```python
from build123d import *

# Parameters (mm, degrees)
SKETCH1_W           = 6
SKETCH1_H           = 20
SKETCH1_R           = 2
BOSS_EXTRUDE1_DEPTH = 3
SKETCH4_R           = 1.5
CUT_EXTRUDE1_DEPTH  = 10
SKETCH5_W           = 0.8
SKETCH5_H           = 4.49496607
CUT_EXTRUDE2_DEPTH  = 7
SKETCH6_R           = 1
CUT_EXTRUDE3_DEPTH  = 7


with BuildPart() as part:
    # Sketch1 → Boss-Extrude1 (new body, symmetric)
    with BuildSketch(Plane.XY):
        with Locations((0, 195)):
            Rectangle(SKETCH1_W, SKETCH1_H)
        with Locations((0, 200)):
            Circle(SKETCH1_R, mode=Mode.SUBTRACT)
    extrude(amount=BOSS_EXTRUDE1_DEPTH, both=True)

    # Sketch3 → Cut-Revolve3 (revolve, cut)
    with BuildSketch(Plane.XY):
        Polygon((-3, 185), (-2.3, 185), (-3, 188.032033112), (-6.917363823, 205), (-6.917363823, 185), align=None)
    revolve(axis=Axis((0, 200, 0), (0, -1, 0)), mode=Mode.SUBTRACT)

    # Sketch4 → Cut-Extrude1 (cut)
    with BuildSketch(Plane.XZ.offset(-185)):
        Circle(SKETCH4_R)
    extrude(amount=-CUT_EXTRUDE1_DEPTH, mode=Mode.SUBTRACT)

    # Sketch5 → Cut-Extrude2 (cut, through all)
    with BuildSketch(Plane.XY.offset(3)):
        with Locations((0, 202.752516965)):
            Rectangle(SKETCH5_W, SKETCH5_H)
    extrude(amount=-CUT_EXTRUDE2_DEPTH, mode=Mode.SUBTRACT)

    # Sketch6 → Cut-Extrude3 (cut, through all)
    with BuildSketch(Plane(origin=(3, 0, 0), x_dir=(0, 0, -1), z_dir=(1, 0, 0))):
        with Locations((0, 203)):
            Circle(SKETCH6_R)
    extrude(amount=-CUT_EXTRUDE3_DEPTH, mode=Mode.SUBTRACT)


solid = part.part
```
The listing builds one solid part. Answer for the finished solid, in the listing's coordinates (mm). A direction names the side the tool comes from. Give positions to 0.01 mm unless a question says otherwise; leave off trailing zeros. Order: outer loops, then holes, each group sorted by start corner. A loop starts at its lowest first (then second) coordinate and runs counter-clockwise, first axis right, second up.
1) Consider line 1 along Z through (x, y) = (1.9, 203); line 2 along Z through (x, y) = (0, 191.25); line 3 along X through (y, z) = (200, 0.35). Determine where each line is inside the solid, lowest interval first.
Reported:
line 1: z = -3 to -1, 1 to 3
line 2: z = -3 to -1.5, 1.5 to 3
line 3: x = -3 to -2, 2 to 3
2) Find section A-A on y = 203. Write down the section's boundary in (x, z), then the cut area to 3 significant figures.
Reported:
outline: (-3, -3) - (-0.4, -3) - (-0.4, -1) - (-3, -1) - close; (-3, 1) - (-0.4, 1) - (-0.4, 3) - (-3, 3) - close; (0.4, -3) - (3, -3) - (3, -1) - (0.4, -1) - close; (0.4, 1) - (3, 1) - (3, 3) - (0.4, 3) - close
area: 20.8 mm2
3) Find section C-C on y = 194. Write down the section's boundary in (x, z), then the cut area to 3 significant figures.
Reported:
outline: (-3, -3) - (3, -3) - (3, 3) - (-3, 3) - close; hole circle Ø3 at (0, 0)
area: 28.9 mm2
4) Find section B-B on y = 200. Write down the section's boundary in (x, z).
Reported:
outline: (-3, -3) - (-2, -3) - (-2, 3) - (-3, 3) - close; (2, -3) - (3, -3) - (3, 3) - (2, 3) - close
5) For faces 5 (the face through (2, 205, 0)), 6 (the face through (0.4, 204, 1)), 7 (the face through (0, 195, 0)), determine the directions among +Z, -Z, +X, -X, +Y, -Y from which every point of the face is accessible in a straight line to the end or side of a thin tool.
Reported:
face 5: +Z, -Z, +X, -X, +Y
face 6: +Z, -Z, +Y
face 7: -Y
6) Find section D-D on x = 1.75. Give the number of separate pieces and of enclosed holes in the cut face, then the cut area to 3 significant figures.
Reported:
separate pieces: 2
enclosed holes: 1
area: 97.9 mm2
7) Determine the mould class of faces 1 (the face through (3, 196, 0)), 2 (the face through (0, 197, -3)), 3 (the face through (-0.4, 204, 1)), 4 (the face through (-3, 196, 0)) for opening direction X: pulls with the +X half, pulls with the -X half, needs draft (parallel to the pull), parting line crosses it, or undercut.
Reported:
face 1: pulls with the +X half
face 2: needs draft
face 3: undercut
face 4: pulls with the -X half
8) Given P1, Ø1.5, axis at x = 0, z = 0, coming from the -Y side, flat-ended and moving along its own axis, determine where the tip first touches the part or whether it passes through.
Reported:
P1: stops at y = 195
